Here's how the part is built. I have some questions about the finished solid (model axes, mm). A direction names the side the tool comes from. Coordinates: 2 decimals unless noted, no trailing zeros. Loops run counter-clockwise (first coordinate to the right, second up) from the corner with the lowest first, then second, coordinate; pieces in that order, holes last. Notation, with made-up numbers: (38.5, -23.5) -> (75.5, -23.5) arc R12 cw to (75.5, -11.5) -> close; hole circle Ø5 at (21.5, 65.25). An arc over 180 degrees is marked (long way). Answer as a JSON object with one key per item and string values. Group by question number.
Q1. I'm going to push flat-ended pins straight in: pin 1 (2 mm diameter, centred on x = 62, y = -10.5, fed in from +Z); pin 2 (10 mm diameter, centred on x = 51, y = -29, fed in from -Z); pin 3 (6 mm diameter, centred on x = 47, y = 3.5, fed in from +Z). Where does each tip first touch, or does it pass through?
Q2. Thinking about a two-plate mould opening in Y: for faces 1 (the cylindrical face through (0.558, 6.439, 95.262)), 2 (the flat face through (85, 0, -38)), 3 (the flat face through (2, 12.7, -2)), which applies, released by +Y, released by -Y, zero draft, split by the parting line, or undercut?
Q3. On a 3-axis mill with a long thin cutter (end or side, diameter ignored), from which of +Z, -Z, +X, -X, +Y, -Y can I reach the whole of each face in a straight line? I mean faces 4 (the cylindrical face through (-48.794, -42.035, -6.406)), 5 (the cylindrical face through (97.477, 6.439, 66.089)). Say none if no direction works.
Q4. I want a section at A-A on x = 0. Count the separate pieces of the cut face and the enclosed holes in it, then the cut area to 3 significant figures.
Q5. I need wall thicknesses on line 1 (Z direction, x = -3, y = 5); line 2 (X direction, y = 3.5, z = -107.95); line 3 (Y direction, x = -98, z = 27). Which ranges of each line are inside material? Lowest first, please.
Q6. I want a section at D-D on z = -107.95. Write out the boundary of the cut face in (x, y).
```python
from build123d import *

# Parameters (mm, degrees)
SKETCH1_R           = 127
BOSS_EXTRUDE1_DEPTH = 12.7
SKETCH2_R           = 12.7
CUT_EXTRUDE1_DEPTH  = 12.7
SKETCH3_R           = 88.9
BOSS_EXTRUDE2_DEPTH = 39.6875
CHAMFER2_SIZE       = 39.6875
SKETCH4_R           = 49.2125
BOSS_EXTRUDE3_DEPTH = 4.7625


with BuildPart() as part:
    # Sketch1 → Boss-Extrude1 (new body)
    with BuildSketch(Plane(origin=(0, 0, 0), x_dir=(1, 0, 0), z_dir=(0, 1, 0))):
        with Locations(Location((0, 0, 0), (0, 0, 270))):
            Circle(SKETCH1_R)
    extrude(amount=BOSS_EXTRUDE1_DEPTH)

    # Sketch2 → Cut-Extrude1 (cut)
    with BuildSketch(Plane(origin=(0, 12.7, 0), x_dir=(1, 0, 0), z_dir=(0, 1, 0))):
        with Locations(Location((0, 107.95, 0), (0, 0, 270))):
            Circle(SKETCH2_R)
        with Locations(Location((0, -107.95, 0), (0, 0, 270))):
            Circle(SKETCH2_R)
        with Locations(Location((93.6625, -53.975, 0), (0, 0, 270))):
            Circle(SKETCH2_R)
        with Locations(Location((93.6625, 53.975, 0), (0, 0, 270))):
            Circle(SKETCH2_R)
        with Locations(Location((-93.6625, 53.975, 0), (0, 0, 270))):
            Circle(SKETCH2_R)
        with Locations(Location((-93.6625, -53.975, 0), (0, 0, 270))):
            Circle(SKETCH2_R)
    extrude(amount=-CUT_EXTRUDE1_DEPTH, mode=Mode.SUBTRACT)

    # Sketch3 → Boss-Extrude2 (add)
    with BuildSketch(Plane(origin=(0, 0, 0), x_dir=(-1, 0, 0), z_dir=(0, -1, 0))):
        with Locations(Location((0, 0, 0), (0, 0, 270))):
            Circle(SKETCH3_R)
    extrude(amount=BOSS_EXTRUDE2_DEPTH)

    # Chamfer2
    chamfer2_edges = [part.edges().sort_by_distance(p)[0] for p in [
        (0, -39.6875, -88.9),
    ]]
    chamfer(chamfer2_edges, length=CHAMFER2_SIZE - 0.0001)  # a hair under: the kernel refuses the full size

    # Sketch4 → Boss-Extrude3 (add)
    with BuildSketch(Plane.XZ.offset(39.6875)):
        with Locations(Location((0, 0, 0), (0, 0, 90))):
            Circle(SKETCH4_R)
    extrude(amount=BOSS_EXTRUDE3_DEPTH)


solid = part.part
```
Result set:
{
 "1": {"pin 1": "stops at z = 50.03", "pin 2": "stops at z = -42.18", "pin 3": "stops at z = 119.13"},
 "2": {"face 1": "zero draft", "face 2": "released by -Y", "face 3": "released by +Y"},
 "3": {"face 4": "-Y", "face 5": "+Y, -Y"},
 "4": {"separate pieces": "3", "enclosed holes": "0", "area": "8,530 mm²"},
 "5": {"line 1": "z = -126.96 to -120.29, -95.61 to 95.61, 120.29 to 126.96", "line 2": "x = -66.9 to -12.7, 12.7 to 66.9", "line 3": "y = 0 to 12.7"},
 "6": {"outline": "(-66.9, 0) -> (-12.7, 0) -> (-12.7, 12.7) -> (-66.9, 12.7) -> close; (12.7, 0) -> (66.9, 0) -> (66.9, 12.7) -> (12.7, 12.7) -> close"}
}
